Work out the finished part from the listing and answer in its coordinate system (mm). Face numbers are marked on the shaded views. A direction names the side the tool comes from. Coordinates: 2 decimals unless noted, no trailing zeros. Write each loop counter-clockwise with the first axis right and the second up, starting at its lowest first coordinate (ties: lowest second). Pieces come first, ordered by that corner, then holes. Notation, with made-up numbers: (27, -1.75) - (64, -1.75) arc R6 cw to (64, 8.25) - close; hole circle Ø11 at (-12.75, -12.75). An arc over 180 degrees is marked (long way). Use a Markdown table: item, result. Add a question column.
(1) Given pin 1 Ø6.5 at (x, z) = (7.5, 6) entering from -Y; pin 2 Ø1.6 at (x, z) = (5, 45.5) entering from +Y; pin 3 Ø3 at (x, z) = (16.5, -45.5) entering from +Y; pin 4 Ø6.5 at (x, z) = (4.5, 46.5) entering from +Y, each flat-ended and moving along its own axis, determine where each tip first touches the part or whether it passes through.
(2) A tool of negligible diameter and unlimited length cuts with its end or side. For the marked faces 1 and 2, from which of +Z, -Z, +X, -X, +Y, -Y can it reach the whole face along a straight path? Write none if from no direction.
(3) Find the intervals of material crossed by line 1 (X direction, y = 4.7, z = -46.5); line 2 (X direction, y = 0.9, z = 46.5); line 3 (Z direction, x = 5.75, y = 4.5), in increasing order. Write a range as from..to.
(4) The part is cut by section A-A, the plane z = -46.5. Give the vertices of the cut face in (x, y), then the cut area to 3 significant figures.
(5) For a pull along Z with two mould halves and no side action, classify the marked faces 3, 4, 5 and 6 as released by +Z, released by -Z, zero draft, split by the parting line, or undercut.
(6) The part is cut by section B-B, the plane x = 10.5. State how many separate pieces and enclosed holes the cut face has, then the cut area to 3 significant figures.
(7) The part is cut by section C-C, the plane z = 46.5. Give the vertices of the cut face in (x, y), then the cut area to 3 significant figures.
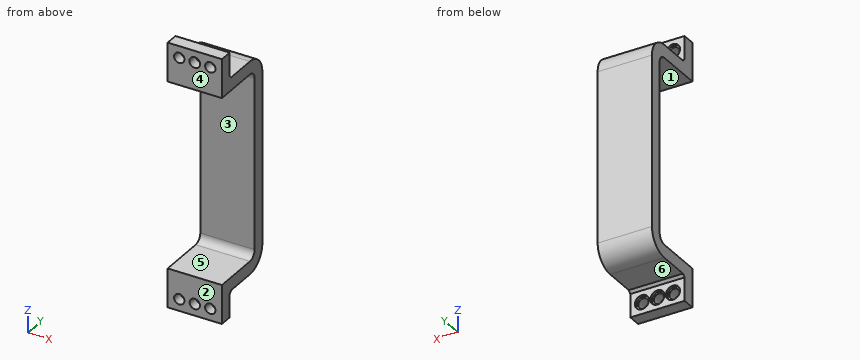
from build123d import *

# Parameters (mm, degrees)
SALIENTE_EXTRUIR1_DEPTH = 21
CROQUIS2_R              = 2.75
CORTAR_EXTRUIR1_DEPTH   = 22
CROQUIS3_R              = 2
CROQUIS3_R_2            = 2.070321152
CROQUIS3_R_3            = 1.933403805
CORTAR_EXTRUIR3_DEPTH   = 22
CROQUIS5_R              = 1.933403805
CROQUIS5_R_2            = 2.015312249
CORTAR_EXTRUIR4_DEPTH   = 22


with BuildPart() as part:
    # Croquis1 → Saliente-Extruir1 (new body)
    with BuildSketch(Plane(origin=(0, 0, 0), x_dir=(0, 0, -1), z_dir=(1, 0, 0))):
        with BuildLine():
            Line((-51, 0), (-36, 0))
            Line((-36, 0), (-36, 18))
            ThreePointArc((-36, 18), (-35.121320344, 20.121320344), (-33, 21))
            Line((-33, 21), (33, 21))
            ThreePointArc((33, 21), (35.121320344, 20.121320344), (36, 18))
            Line((36, 18), (36, 0))
            Line((36, 0), (51, 0))
            Line((51, 0), (51, 5))
            Line((51, 5), (42, 5))
            Line((42, 5), (41, 6))
            Line((41, 6), (41, 18))
            ThreePointArc((41, 18), (38.656854249, 23.656854249), (33, 26))
            Line((33, 26), (-33, 26))
            ThreePointArc((-33, 26), (-38.656854249, 23.656854249), (-41, 18))
            Line((-41, 18), (-41, 6))
            Line((-41, 6), (-42, 5))
            Line((-42, 5), (-51, 5))
            Line((-51, 5), (-51, 0))
        make_face()
    extrude(amount=SALIENTE_EXTRUIR1_DEPTH)

    # Croquis2 → Cortar-Extruir1 (cut)
    with BuildSketch(Plane(origin=(0, 26, 0), x_dir=(1, 0, 0), z_dir=(0, 1, 0))):
        with Locations(Location((10.5, 46.5, 0), (0, 0, 270))):
            Circle(CROQUIS2_R)
        with Locations(Location((16.5, 46.5, 0), (0, 0, 270))):
            Circle(CROQUIS2_R)
        with Locations(Location((4.5, 46.5, 0), (0, 0, 270))):
            Circle(CROQUIS2_R)
        with Locations(Location((16.5, -46.5, 0), (0, 0, 90))):
            Circle(CROQUIS2_R)
        with Locations(Location((10.5, -46.5, 0), (0, 0, 90))):
            Circle(CROQUIS2_R)
        with Locations(Location((4.5, -46.5, 0), (0, 0, 90))):
            Circle(CROQUIS2_R)
    extrude(amount=-CORTAR_EXTRUIR1_DEPTH, mode=Mode.SUBTRACT)

    # Croquis3 → Cortar-Extruir3 (cut)
    # profile 1 of 6: a face of its own
    with BuildSketch(Plane(origin=(0, 4, 0), x_dir=(1, 0, 0), z_dir=(0, 1, 0))):
        with Locations(Location((4.5, 46.5, 0), (0, 0, 270))):
            Circle(CROQUIS3_R)
    # profile 2 of 6: a face of its own
    with BuildSketch(Plane(origin=(0, 4, 0), x_dir=(1, 0, 0), z_dir=(0, 1, 0))):
        with Locations(Location((10.5, 46.5, 0), (0, 0, 270))):
            Circle(CROQUIS3_R)
    # profile 3 of 6: a face of its own
    with BuildSketch(Plane(origin=(0, 4, 0), x_dir=(1, 0, 0), z_dir=(0, 1, 0))):
        with Locations(Location((16.5, 46.5, 0), (0, 0, 270))):
            Circle(CROQUIS3_R)
    # profile 4 of 6: a face of its own
    with BuildSketch(Plane(origin=(0, 4, 0), x_dir=(1, 0, 0), z_dir=(0, 1, 0))):
        with Locations(Location((10.5, -46.5, 0), (0, 0, 270))):
            Circle(CROQUIS3_R_2)
        with Locations(Location((10.5, -46.5, 0), (0, 0, 270))):
            Circle(CROQUIS3_R, mode=Mode.SUBTRACT)
    # profile 5 of 6: a face of its own
    with BuildSketch(Plane(origin=(0, 4, 0), x_dir=(1, 0, 0), z_dir=(0, 1, 0))):
        with Locations(Location((16.5, -46.5, 0), (0, 0, 270))):
            Circle(CROQUIS3_R)
        with Locations(Location((16.5, -46.5, 0), (0, 0, 270))):
            Circle(CROQUIS3_R_3, mode=Mode.SUBTRACT)
    # profile 6 of 6: a face of its own
    with BuildSketch(Plane(origin=(0, 4, 0), x_dir=(1, 0, 0), z_dir=(0, 1, 0))):
        with Locations(Location((4.5, -46.5, 0), (0, 0, 270))):
            Circle(CROQUIS3_R)
        with Locations(Location((4.5, -46.5, 0), (0, 0, 270))):
            Circle(CROQUIS3_R_3, mode=Mode.SUBTRACT)
    extrude(amount=-CORTAR_EXTRUIR3_DEPTH, mode=Mode.SUBTRACT)


with BuildPart() as cortar_extruir3_piece_1:
    # of the separate pieces the step leaves, piece 1, a body of its own (cortar_extruir3_pieces)
    add(part.part.solids().sort_by_distance((0, 18, 41))[0])


with BuildPart() as cortar_extruir3_piece_2:
    # of the separate pieces the step leaves, piece 2, a body of its own (cortar_extruir3_pieces)
    add(part.part.solids().sort_by_distance((10.5, 0, 48.5))[0])


with BuildPart() as cortar_extruir3_piece_3:
    # of the separate pieces the step leaves, piece 3, a body of its own (cortar_extruir3_pieces)
    add(part.part.solids().sort_by_distance((4.5, 0, 48.433403805))[0])


with BuildPart() as cortar_extruir3_piece_4:
    # of the separate pieces the step leaves, piece 4, a body of its own (cortar_extruir3_pieces)
    add(part.part.solids().sort_by_distance((16.5, 0, 48.433403805))[0])


with BuildPart() as cortar_extruir4_tool:
    # Croquis5 → Cortar-Extruir4 (new body)
    with BuildSketch(Plane(origin=(0, 4, 0), x_dir=(1, 0, 0), z_dir=(0, 1, 0))):
        with Locations((4.5, -46.5)):
            Circle(CROQUIS5_R)
        with Locations((10.5, -46.5)):
            Circle(CROQUIS5_R_2)
        with Locations((16.5, -46.5)):
            Circle(CROQUIS5_R)
    extrude(amount=-CORTAR_EXTRUIR4_DEPTH)


with BuildPart() as cortar_extruir3_piece_2_1:
    add(cortar_extruir3_piece_2.part)

    # Cortar-Extruir4: cut by cortar_extruir4_tool
    add(cortar_extruir4_tool.part, mode=Mode.SUBTRACT)


with BuildPart() as cortar_extruir3_piece_3_1:
    add(cortar_extruir3_piece_3.part)

    # Cortar-Extruir4: cut by cortar_extruir4_tool
    add(cortar_extruir4_tool.part, mode=Mode.SUBTRACT)


with BuildPart() as cortar_extruir3_piece_4_1:
    add(cortar_extruir3_piece_4.part)

    # Cortar-Extruir4: cut by cortar_extruir4_tool
    add(cortar_extruir4_tool.part, mode=Mode.SUBTRACT)


solid = cortar_extruir3_piece_1.part
Model answer:
| question | item | result |
|---|---|---|
| 1 | pin 1 | y = 21 |
| 1 | pin 2 | through |
| 1 | pin 3 | y = 4 |
| 1 | pin 4 | y = 5 |
| 2 | face 1 | +X, -X, -Y |
| 2 | face 2 | +Z, -Z, +X, -X, -Y |
| 3 | line 1 | 0..1.75, 7.25..7.75, 13.25..13.75, 19.25..21 |
| 3 | line 2 | 0..2.5, 6.5..8.43, 12.57..14.5, 18.5..21 |
| 3 | line 3 | -51..-48.95, -44.05..-36, 36..44.05, 48.95..51 |
| 4 | outline | (0, 0) - (2.5, 0) - (2.5, 4) - (1.75, 4) - (1.75, 5) - (0, 5) - close; (6.5, 0) - (8.5, 0) - (8.5, 4) - (7.75, 4) - (7.75, 5) - (7.25, 5) - (7.25, 4) - (6.5, 4) - close; (12.5, 0) - (14.5, 0) - (14.5, 4) - (13.75, 4) - (13.75, 5) - (13.25, 5) - (13.25, 4) - (12.5, 4) - close; (18.5, 0) - (21, 0) - (21, 5) - (19.25, 5) - (19.25, 4) - (18.5, 4) - close |
| 4 | area | 40.5 mm^2 |
| 5 | face 3 | undercut |
| 5 | face 4 | zero draft |
| 5 | face 5 | undercut |
| 5 | face 6 | released by -Z |
| 6 | separate pieces | 3 |
| 6 | enclosed holes | 0 |
| 6 | area | 654 mm^2 |
| 7 | outline | (0, 0) - (2.5, 0) - (2.5, 4) - (1.75, 4) - (1.75, 5) - (0, 5) - close; (6.5, 0) - (8.43, 0) - (8.43, 4) - (7.75, 4) - (7.75, 5) - (7.25, 5) - (7.25, 4) - (6.5, 4) - close; (12.57, 0) - (14.5, 0) - (14.5, 4) - (13.75, 4) - (13.75, 5) - (13.25, 5) - (13.25, 4) - (12.57, 4) - close; (18.5, 0) - (21, 0) - (21, 5) - (19.25, 5) - (19.25, 4) - (18.5, 4) - close |
| 7 | area | 39.9 mm^2 |
